```python
from build123d import *

# Parameters (mm, degrees)
SKETCH1_W           = 150
SKETCH1_H           = 55
SKETCH1_R           = 12.5
BOSS_EXTRUDE1_DEPTH = 4
SKETCH2_R           = 1.4
CUT_EXTRUDE1_DEPTH  = 80.982810653
SKETCH3_R           = 2.5
CUT_EXTRUDE3_DEPTH  = 2
FILLET1_R           = 10
SKETCH4_W           = 30
SKETCH4_H           = 12.357308998
CUT_EXTRUDE4_DEPTH  = 80.982810653


with BuildPart() as part:
    # Sketch1 → Boss-Extrude1 (new body)
    with BuildSketch(Plane(origin=(0, 0, 0), x_dir=(1, 0, 0), z_dir=(0, 1, 0))):
        Rectangle(SKETCH1_W, SKETCH1_H)
        with Locations(Location((-50, 0, 0), (0, 0, 270))):
            Circle(SKETCH1_R, mode=Mode.SUBTRACT)
        with Locations(Location((50, 0, 0), (0, 0, 270))):
            Circle(SKETCH1_R, mode=Mode.SUBTRACT)
    extrude(amount=BOSS_EXTRUDE1_DEPTH)

    # Sketch2 → Cut-Extrude1 (cut, through all)
    with BuildSketch(Plane(origin=(0, 4, 0), x_dir=(1, 0, 0), z_dir=(0, 1, 0))):
        with Locations(Location((30.514428415, 11.25, 0), (0, 0, 270))):
            Circle(SKETCH2_R)
        with Locations(Location((69.485571585, 11.25, 0), (0, 0, 270))):
            Circle(SKETCH2_R)
        with Locations(Location((69.485571585, -11.25, 0), (0, 0, 270))):
            Circle(SKETCH2_R)
        with Locations(Location((30.514428415, -11.25, 0), (0, 0, 270))):
            Circle(SKETCH2_R)
        with Locations(Location((50, -22.5, 0), (0, 0, 270))):
            Circle(SKETCH2_R)
    cut_extrude1 = extrude(amount=-CUT_EXTRUDE1_DEPTH, mode=Mode.SUBTRACT)

    # Sketch3 → Cut-Extrude3 (cut)
    with BuildSketch(Plane(origin=(0, 4, 0), x_dir=(1, 0, 0), z_dir=(0, 1, 0))):
        with Locations(Location((30.514428415, 11.25, 0), (0, 0, 270))):
            Circle(SKETCH3_R)
        with Locations(Location((30.514428415, -11.25, 0), (0, 0, 270))):
            Circle(SKETCH3_R)
        with Locations(Location((50, -22.5, 0), (0, 0, 270))):
            Circle(SKETCH3_R)
        with Locations(Location((69.485571585, -11.25, 0), (0, 0, 270))):
            Circle(SKETCH3_R)
        with Locations(Location((69.485571585, 11.25, 0), (0, 0, 270))):
            Circle(SKETCH3_R)
    cut_extrude3 = extrude(amount=-CUT_EXTRUDE3_DEPTH, mode=Mode.SUBTRACT)

    # Mirror1: Cut-Extrude1, Cut-Extrude3 across plane
    add(cut_extrude1.mirror(Plane(origin=(0, 0, 0), x_dir=(0, 0, 1), z_dir=(1, 0, 0))), mode=Mode.SUBTRACT)
    add(cut_extrude3.mirror(Plane(origin=(0, 0, 0), x_dir=(0, 0, 1), z_dir=(1, 0, 0))), mode=Mode.SUBTRACT)

    # Fillet1
    fillet1_edges = [part.edges().sort_by_distance(p)[0] for p in [
        (-75, 2, -27.5),
        (75, 2, -27.5),
        (75, 2, 27.5),
        (-75, 2, 27.5),
    ]]
    fillet(fillet1_edges, radius=FILLET1_R)

    # Sketch4 → Cut-Extrude4 (cut, through all)
    with BuildSketch(Plane.XZ):
        with Locations((-49.04071088, -21.321345501)):
            Rectangle(SKETCH4_W, SKETCH4_H)
        with Locations((50, -21.321345501)):
            Rectangle(SKETCH4_W, SKETCH4_H)
    extrude(amount=-CUT_EXTRUDE4_DEPTH, mode=Mode.SUBTRACT)


solid = part.part
```
Model file for the job. Use its own axes, mm. A direction names the side the tool comes from. Coordinates: 2 decimals unless noted, no trailing zeros. Loops run counter-clockwise (first coordinate to the right, second up) from the corner with the lowest first, then second, coordinate; pieces in that order, holes last. Notation, with made-up numbers: (-33.5, 82) - (-25.5, 82) arc R32 ccw to (-25.5, 109) - close; hole circle Ø9 at (62, 15.25). An arc over 180 degrees is marked (long way). Write item = value, one per line. Start each with the question number.
Item 1: Saw through at C-C, the plane y = 0.65. State how many separate pieces and enclosed holes the cut face has, then the cut area to 3 significant figures.
Item 2: Wall check: probe 1 along X at (y, z) = (2.15, -4); probe 2 along X at (y, z) = (3.75, -5.5); probe 3 along Z at (x, y) = (51, 3). Give the ranges that are in metal, low to high. Write a range as [from, to].
Item 3: Drop flat-ended pins along their axis: pin 1 Ø2 at (x, y) = (48, 2) entering from -Z; pin 2 Ø2.5 at (x, z) = (-30, 11) entering from +Y; pin 3 Ø2.5 at (x, z) = (69.49, -11.25) entering from -Y. Give the stop position or say it passes through.
Item 4: 3-axis set-ups, long thin cutter, end or side, ignore diameter. For faces 5 (the face through (-64.041, 2, -21)), 6 (the face through (37.797, 1.972, -2.71)), 7 (the face through (-49, 2, 24)): which of +Z, -Z, +X, -X, +Y, -Y reach the whole face in a straight line?
Item 5: Saw through at D-D, the plane z = 22.5. List the corners of the cut face in (x, y), then the cut area to 3 significant figures.
Item 6: Saw through at B-B, the plane x = 50. List the corners of the cut face in (y, z).
Item 7: Saw through at A-A, the plane z = 0. List the corners of the cut face in (x, y), then the cut area to 3 significant figures.
Item 8: Pull direction Z, two halves, no side cores. Call faces 1 (the face through (71.99, 2.03, 24.65)), 2 (the face through (-1, 0, 0)), 3 (the face through (-67, 3, 11)), 4 (the face through (-68, 2, 12)): +Z half, -Z half, draft (parallel to the pull), parting line (faces both ways), or undercut.
Answers:
q1.separate_pieces = 1
q1.enclosed_holes = 12
q1.area = 6,380 mm2
q2.probe_1 = [-75, -61.84], [-38.16, 38.16], [61.84, 75]
q2.probe_2 = [-75, -61.22], [-38.78, 38.78], [61.22, 75]
q2.probe_3 = [-15.14, -12.46], [12.46, 20.21], [24.79, 27.5]
q3.pin_1 = -15.14
q3.pin_2 = 2
q3.pin_3 = through
q4.face_5 = -Z, +Y, -Y
q4.face_6 = +Y, -Y
q4.face_7 = +Y
q5.outline = (-73.66, 0) - (-51.4, 0) - (-51.4, 2) - (-52.5, 2) - (-52.5, 4) - (-73.66, 4) - close; (-48.6, 0) - (48.6, 0) - (48.6, 2) - (47.5, 2) - (47.5, 4) - (-47.5, 4) - (-47.5, 2) - (-48.6, 2) - close; (51.4, 0) - (73.66, 0) - (73.66, 4) - (52.5, 4) - (52.5, 2) - (51.4, 2) - close
q5.area = 558 mm2
q6.outline = (0, -15.14) - (4, -15.14) - (4, -12.5) - (0, -12.5) - close; (0, 12.5) - (4, 12.5) - (4, 20) - (2, 20) - (2, 21.1) - (0, 21.1) - close; (0, 23.9) - (2, 23.9) - (2, 25) - (4, 25) - (4, 27.5) - (0, 27.5) - close
q7.outline = (-75, 0) - (-62.5, 0) - (-62.5, 4) - (-75, 4) - close; (-37.5, 0) - (37.5, 0) - (37.5, 4) - (-37.5, 4) - close; (62.5, 0) - (75, 0) - (75, 4) - (62.5, 4) - close
q7.area = 400 mm2
q8.face_1 = +Z half
q8.face_2 = draft
q8.face_3 = undercut
q8.face_4 = undercut
